The model under review builds one solid part; all positions refer to its coordinate system, in mm. Face numbers are marked on the shaded views. A direction names the side the tool comes from. Round coordinates to 2 decimals unless told otherwise and drop trailing zeros. Order: outer loops, then holes, each group sorted by start corner. A loop starts at its lowest first (then second) coordinate and runs counter-clockwise, first axis right, second up.
1) Machinability: for the marked faces 1, 2 and 3, which of the approach directions +Z, -Z, +X, -X, +Y, -Y give a long, thin tool a straight path to every point of the face, cutting with its end or side? Answer none if there is none.
2) Clearance check with flat-ended pins moving along their axes: P1, Ø6, axis at y = -128.5, z = 31.5, coming from the +X side; P2, Ø0.8, axis at x = 0.5, y = -132, coming from the -Z side. State where each tip first meets the part, or that it passes through.
3) To check wall thickness, follow L1, parallel to X at y = -120, z = 39; L2, parallel to X at y = -100, z = 18; L3, parallel to Z at x = 0.4, y = -132.5. State the ranges of each line that lie inside material, in increasing order.
4) Consider section A-A (z = 44.5). Give the boundary of the cut face in (x, y).
5) Consider section B-B (y = -105.5). Give the boundary of the cut face in (x, z).
6) Consider section C-C (y = -131). Give the boundary of the cut face in (x, z), then the cut area to 3 significant figures.
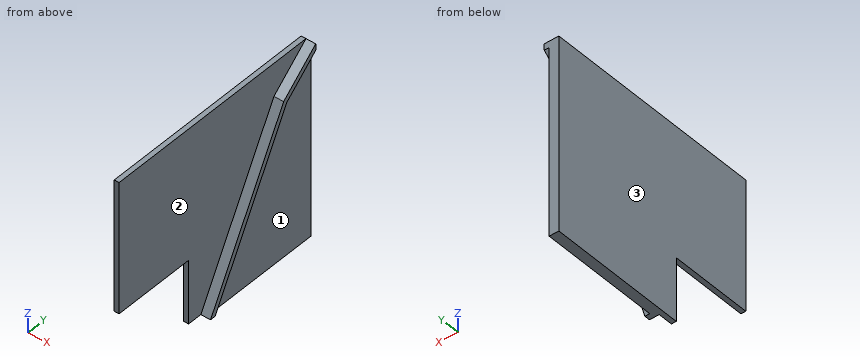
from build123d import *

# Parameters (mm, degrees)
F1_DEPTH = 1
F2_DEPTH = 3
F3_DEPTH = 2


with BuildPart() as f1:
    # F0 (on Right) → F1 (new body)
    with BuildSketch(Plane.YZ):
        Polygon((-91.161479, 53.232064), (-137.161479, 53.232064), (-137.161479, 26.232064), (-127.161479, 26.232064), (-120.057479, 26.232064), (-120.057479, 13.132064), (-117.057479, 13.132064), (-99.057374, 46.433675), align=None)
    extrude(amount=F1_DEPTH)

    # F0 (on Right) → F2 (join)
    with BuildSketch(Plane.YZ):
        Polygon((-91.161479, 51.912471), (-91.161479, 53.232064), (-99.057374, 46.433675), (-117.057479, 13.132064), (-115.920747, 13.132064), (-98.265271, 45.796085), align=None)
    extrude(amount=F2_DEPTH)

    # F0 (on Right) → F3 (join)
    with BuildSketch(Plane.YZ):
        Polygon((-91.161479, 26.232064), (-91.161479, 51.912471), (-98.265271, 45.796085), (-115.920747, 13.132064), (-91.161479, 13.132064), align=None)
    extrude(amount=F3_DEPTH)


solid = f1.part
Answer below:
1. face 1: -Z, +X, +Y
1. face 2: +Z, +X, -Y
1. face 3: +Z, -Z, -X, +Y, -Y
2. P1: stops at x = 1
2. P2: stops at z = 26.23
3. L1: x = 0 to 1
3. L2: x = 0 to 2
3. L3: z = 26.23 to 53.23
4. outline: (0, -137.16) - (1, -137.16) - (1, -100.1) - (3, -100.1) - (3, -98.97) - (2, -98.97) - (2, -91.16) - (0, -91.16) - close
5. outline: (0, 13.13) - (2, 13.13) - (2, 32.41) - (3, 32.41) - (3, 34.51) - (1, 34.51) - (1, 53.23) - (0, 53.23) - close
6. outline: (0, 26.23) - (1, 26.23) - (1, 53.23) - (0, 53.23) - close
6. area: 27.0 mm2
